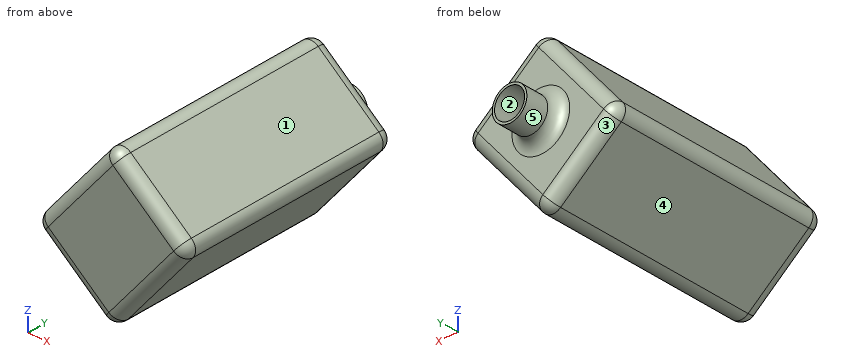
from build123d import *

# Parameters (mm, degrees)
BOSS_EXTRUDE2_DEPTH = 200
BOSS_EXTRUDE3_DEPTH = 200
BOSS_EXTRUDE4_DEPTH = 200
BOSS_EXTRUDE5_REACH = 247.011
SKETCH2_W           = 108.348849956
SKETCH2_H           = 6.424491228
SKETCH2_H_2         = 5.401330914
SKETCH3_R           = 15
SKETCH3_R_2         = 13
BOSS_EXTRUDE6_DEPTH = 30
FILLET4_R           = 10
FILLET5_R           = 10


with BuildPart() as part:
    # Sketch1 → Boss-Extrude2 (new body)
    with BuildSketch(Plane(origin=(0, 0, 0), x_dir=(1, 0, 0), z_dir=(0, 1, 0))):
        Polygon((-0.406350975, 69.787624434), (-68.386407424, 13.920378043), (0.406350975, -69.787624434), (68.386407424, -13.920378043), align=None)
        Polygon((54.311430077, -12.543783452), (-1.782945566, 55.712647086), (-54.311430077, 12.543783452), (1.782945566, -55.712647086), align=None, mode=Mode.SUBTRACT)
    extrude(amount=BOSS_EXTRUDE2_DEPTH)

    # Sketch1_2 → Boss-Extrude3 (add)
    with BuildSketch(Plane(origin=(0, 0, 0), x_dir=(1, 0, 0), z_dir=(0, 1, 0))):
        Polygon((-0.406350975, 69.787624434), (-68.386407424, 13.920378043), (0.406350975, -69.787624434), (68.386407424, -13.920378043), align=None)
        Polygon((54.311430077, -12.543783452), (-1.782945566, 55.712647086), (-54.311430077, 12.543783452), (1.782945566, -55.712647086), align=None, mode=Mode.SUBTRACT)
    extrude(amount=BOSS_EXTRUDE3_DEPTH)

    # Sketch1_4 → Boss-Extrude4 (add)
    with BuildSketch(Plane(origin=(0, 0, 0), x_dir=(1, 0, 0), z_dir=(0, 1, 0))):
        Polygon((-0.406350975, 69.787624434), (-68.386407424, 13.920378043), (0.406350975, -69.787624434), (68.386407424, -13.920378043), align=None)
        Polygon((54.311430077, -12.543783452), (-1.782945566, 55.712647086), (-54.311430077, 12.543783452), (1.782945566, -55.712647086), align=None, mode=Mode.SUBTRACT)
    extrude(amount=BOSS_EXTRUDE4_DEPTH)

    # Sketch2 → Boss-Extrude5 (add, up to next)
    with BuildSketch(Plane(origin=(33.990028225, 0, -27.933623196), x_dir=(-0.6349191378309257, 0, -0.7725785969181609), z_dir=(0.772578596918161, 0, -0.6349191378309257)), mode=Mode.PRIVATE) as boss_extrude5_sk1:
        with Locations((0, 3.212245614)):
            Rectangle(SKETCH2_W, SKETCH2_H)
    boss_extrude5_tool1 = extrude(boss_extrude5_sk1.sketch, amount=-BOSS_EXTRUDE5_REACH, mode=Mode.PRIVATE) - part.part
    # Sketch2 → Boss-Extrude5 (add, up to next)
    with BuildSketch(Plane(origin=(33.990028225, 0, -27.933623196), x_dir=(-0.6349191378309257, 0, -0.7725785969181609), z_dir=(0.772578596918161, 0, -0.6349191378309257)), mode=Mode.PRIVATE) as boss_extrude5_sk2:
        with Locations((0, 197.299334543)):
            Rectangle(SKETCH2_W, SKETCH2_H_2)
    boss_extrude5_tool2 = extrude(boss_extrude5_sk2.sketch, amount=-BOSS_EXTRUDE5_REACH, mode=Mode.PRIVATE) - part.part
    add(boss_extrude5_tool1.solids().sort_by_distance((33.990028, 3.212246, -27.933623))[0])
    add(boss_extrude5_tool2.solids().sort_by_distance((33.990028, 197.299335, -27.933623))[0])

    # Sketch3 → Boss-Extrude6 (add)
    with BuildSketch(Plane(origin=(0, 200, 0), x_dir=(1, 0, 0), z_dir=(0, 1, 0))):
        with Locations(Location((0, 0, 0), (0, 0, 270))):
            Circle(SKETCH3_R)
        with Locations(Location((0, 0, 0), (0, 0, 270))):
            Circle(SKETCH3_R_2, mode=Mode.SUBTRACT)
    extrude(amount=BOSS_EXTRUDE6_DEPTH)

    # Fillet4
    fillet4_edges = [part.edges().sort_by_distance(p)[0] for p in [
        (0, 200, -15),
    ]]
    fillet(fillet4_edges, radius=FILLET4_R)

    # Fillet5
    fillet5_edges = [part.edges().sort_by_distance(p)[0] for p in [
        (-33.990028225, 200, 27.933623196),
        (34.396379199, 200, 41.854001238),
        (33.990028225, 200, -27.933623196),
        (34.396379199, 0, 41.854001238),
        (-33.990028225, 0, 27.933623196),
        (-34.396379199, 0, -41.854001238),
        (33.990028225, 0, -27.933623196),
        (68.386407424, 100, 13.920378043),
        (0.406350975, 100, 69.787624434),
        (-68.386407424, 100, -13.920378043),
        (-0.406350975, 100, -69.787624434),
        (-34.396379199, 200, -41.854001238),
    ]]
    fillet(fillet5_edges, radius=FILLET5_R)


solid = part.part
Geometry: final body of the model. Coordinates: model frame, mm. Face numbers are marked on the shaded views. A direction names the side the tool comes from. Give positions to 0.01 mm unless a question says otherwise; leave off trailing zeros. Write each loop counter-clockwise with the first axis right and the second up, starting at its lowest first coordinate (ties: lowest second). Pieces come first, ordered by that corner, then holes. Notation, with made-up numbers: (-3.5, 83) -> (46.5, 83) arc R10 cw to (46.5, 97) -> close; hole circle Ø4 at (20.5, 5). An arc over 180 degrees is marked (long way). Answer as a JSON object with one key per item and string values.
1. Access query for the marked faces 4 and 5. Directions: +Z, -Z, +X, -X, +Y, -Y. A direction counts if a zero-diameter tool reaches every point of the face in a straight line with its end or side. Return the directions, or none.
Ans:
{"face 4": "-Z, -X, +Y, -Y", "face 5": "+Y"}
2. Mould query, pull axis Z, two halves, no side actions, for the marked faces 1, 2 and 3. Classes: pulls with the +Z half, pulls with the -Z half, needs draft (parallel to the pull), parting line crosses it, or undercut.
Ans:
{"face 1": "pulls with the +Z half", "face 2": "undercut", "face 3": "pulls with the -Z half"}
3. Cut plane A-A on y = 132.5. Output: boundary loops of the cut face in (x, z), and give its area (3 significant figures).
Ans:
{"outline": "(-62.04, -6.19) arc R10 ccw to (-60.66, -20.27) -> (-8.13, -63.44) arc R10 ccw to (5.94, -62.06) -> (62.04, 6.19) arc R10 ccw to (60.66, 20.27) -> (8.13, 63.44) arc R10 ccw to (-5.94, 62.06) -> close; hole (-54.31, -12.54) -> (-1.78, -55.71) -> (54.31, 12.54) -> (1.78, 55.71) -> close", "area": "3,440 mm^2"}
4. Contact query for flat-ended pins moving along their axis: pin 1 (8 mm diameter, centred on x = -50.5, y = 62, fed in from +Z); pin 2 (10 mm diameter, centred on y = 61.5, z = -2, fed in from +X); pin 3 (1.5 mm diameter, centred on y = 44, z = 28, fed in from -X). Output: stop coordinate, or through.
Ans:
{"pin 1": "stops at z = 12.71", "pin 2": "stops at x = 59.41", "pin 3": "stops at x = -34.55"}
5. Ray query, probe 1 along X at (y, z) = (214.75, 0); probe 2 along Y at (x, z) = (-12, 6); probe 3 along Y at (x, z) = (29, 17.5). Return the intervals inside material, ascending. Write a range as from..to.
Ans:
{"probe 1": "x = -15..-13, 13..15", "probe 2": "y = 0..6.42, 194.6..230", "probe 3": "y = 0..6.42, 194.6..200"}
